from build123d import *

# Parameters (mm, degrees)
ESQUISSE10_R       = 4.024
ESQUISSE10_R_2     = 1.5
BOSS_EXTRU_1_DEPTH = 3


with BuildPart() as part:
    # Esquisse10 → Boss.-Extru.1 (new body)
    with BuildSketch(Plane(origin=(0, 0, 0), x_dir=(1, 0, 0), z_dir=(0, 1, 0))):
        with BuildLine():
            Line((-4.472135955, 4), (-40.527864045, 4))
            ThreePointArc((-40.527864045, 4), (-47.140932539, 5.605034154), (-51, 0))
            Line((-51, 0), (-54.677584007, -3.462895596))
            ThreePointArc((-54.677584007, -3.462895596), (-58.082929496, -13.426321088), (-48.442388155, -9.192388155))
            Line((-48.442388155, -9.192388155), (-45, -6))
            ThreePointArc((-45, -6), (-42.550510257, -5.477225575), (-40.527864045, -4))
            Line((-40.527864045, -4), (-4.472135955, -4))
            ThreePointArc((-4.472135955, -4), (6, 0), (-4.472135955, 4))
        make_face()
        with Locations((-54.192388155, -9.192388155)):
            Circle(ESQUISSE10_R, mode=Mode.SUBTRACT)
        with Locations((-45, 0)):
            Circle(ESQUISSE10_R_2, mode=Mode.SUBTRACT)
        Circle(ESQUISSE10_R_2, mode=Mode.SUBTRACT)
    extrude(amount=BOSS_EXTRU_1_DEPTH)


solid = part.part
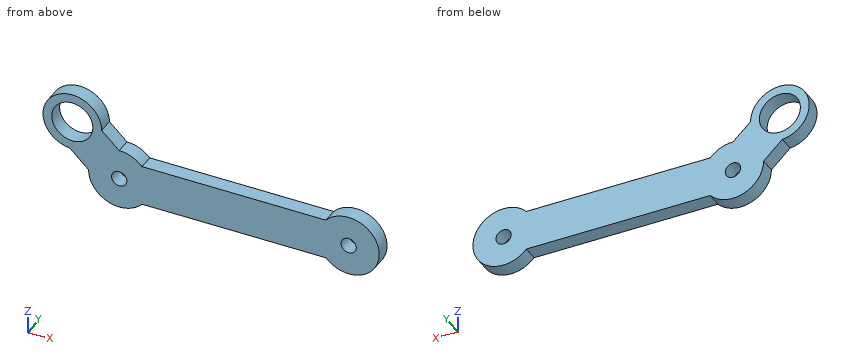
The listing builds one solid part. Answer for the finished solid, in the listing's coordinates (mm). Give positions to 0.01 mm unless a question says otherwise; leave off trailing zeros. Order: outer loops, then holes, each group sorted by start corner. A loop starts at its lowest first (then second) coordinate and runs counter-clockwise, first axis right, second up. Notation, with made-up numbers: (24, 50.25) - (29, 50.25) arc R13 ccw to (29, 72.25) - close; hole circle Ø11 at (-15.75, 40). An arc over 180 degrees is marked (long way). Answer as CSV lines item,"result".
Q1. Each of these flat-tipped pins is pushed along its axis until it touches: pin 1 Ø1 at (y, z) = (2.5, -3.5) entering from +X; pin 2 Ø12 at (x, z) = (-52, 7.5) entering from -Y; pin 3 Ø2.5 at (x, z) = (-45, 0) entering from -Y. Where does it stop, or does it pass through?
Answer key:
pin 1,"stops at x = 5.2"
pin 2,"stops at y = 0"
pin 3,"passes through"
Q2. Straight lines are drawn through the part: L1, parallel to X at y = 1.25, z = 0; L2, parallel to Z at x = -45, y = 1.7; L3, parallel to X at y = 1, z = -0.75. For each, find the intervals that lie inside material, in ascending order.
Answer key:
L1,"x = -51 to -46.5, -43.5 to -1.5, 1.5 to 6"
L2,"z = -6 to -1.5, 1.5 to 6"
L3,"x = -50.95 to -46.3, -43.7 to -1.3, 1.3 to 5.95"
Q3. A cutting plane is placed at D-D, the plane x = -16.5. Determine the outline of the cut face in (y, z).
Answer key:
outline,"(0, -4) - (3, -4) - (3, 4) - (0, 4) - close"
Q4. A cutting plane is placed at B-B, the plane y = 1.75. Determine the outline of the cut face in (x, z).
Answer key:
outline,"(-54.68, 3.46) - (-51, 0) arc R6 ccw to (-40.53, -4) - (-4.47, -4) arc R6 ccw (long way) to (-4.47, 4) - (-40.53, 4) arc R6 ccw to (-45, 6) - (-48.44, 9.19) arc R5.75 ccw (long way) to start; hole circle Ø8.05 at (-54.19, 9.19); hole circle Ø3 at (-45, 0); hole circle Ø3 at (0, 0)"
Q5. A cutting plane is placed at C-C, the plane x = -54. Determine the outline of the cut face in (y, z), and give its area (3 significant figures).
Answer key:
outline,"(0, 2.82) - (3, 2.82) - (3, 5.17) - (0, 5.17) - close; (0, 13.21) - (3, 13.21) - (3, 14.94) - (0, 14.94) - close"
area,"12.2 mm^2"
Q6. A cutting plane is placed at A-A, the plane x = 0. Determine the outline of the cut face in (y, z), and give its area (3 significant figures).
Answer key:
outline,"(0, -6) - (3, -6) - (3, -1.5) - (0, -1.5) - close; (0, 1.5) - (3, 1.5) - (3, 6) - (0, 6) - close"
area,"27.0 mm^2"
